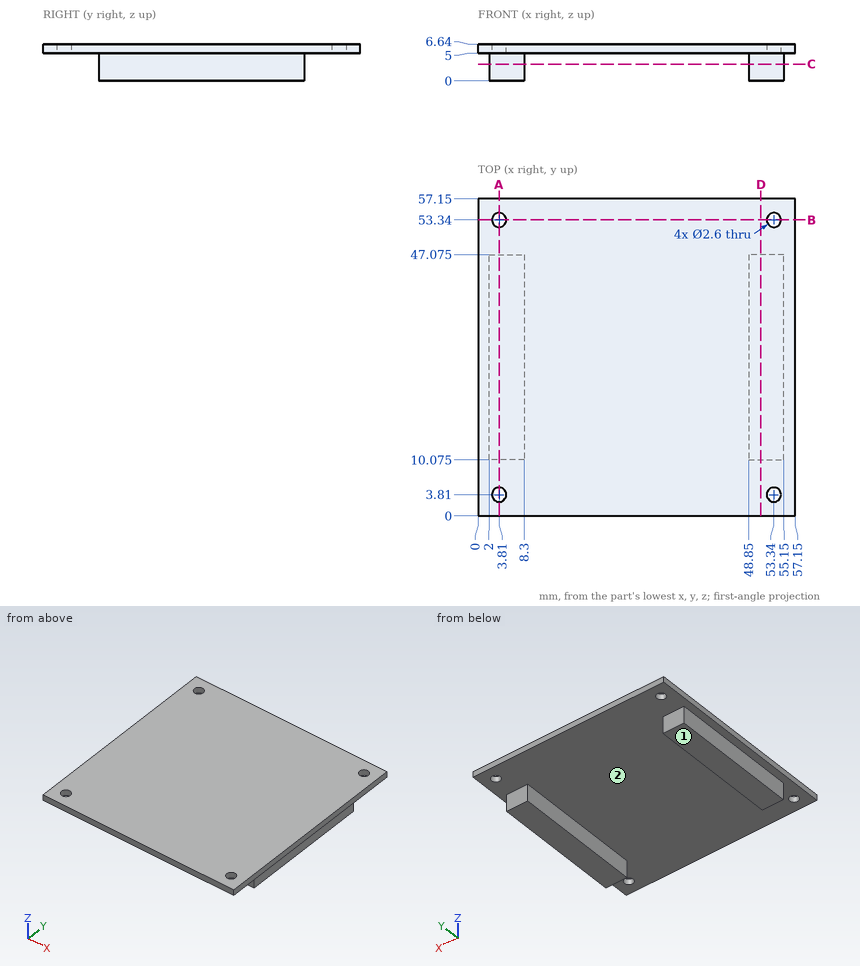
Source: three-view drawing plus pictorial views. Frame: mm from the lowest corner of the part. Round coordinates to 2 decimals unless told otherwise and drop trailing zeros. Loops run counter-clockwise (first coordinate to the right, second up) from the corner with the lowest first, then second, coordinate; pieces in that order, holes last.
1. Ray query, L1, parallel to Y at x = 53.34, z = 6.15; L2, parallel to X at y = 23, z = 3; L3, parallel to Y at x = 54, z = 5.5. Return the intervals inside material, ascending.
2. Section query A-A on x = 3.81. Output: boundary loops of the cut face in (y, z) (3 decimals).
3. Section query B-B on y = 53.34. Output: boundary loops of the cut face in (x, z).
4. Section query C-C on z = 3. Output: boundary loops of the cut face in (x, y) (3 decimals).
5. Contact query for flat-ended pins moving along their axis: pin 1 (2.5 mm diameter, centred on x = 51, z = 3.5, fed in from +Y) (3 decimals); pin 2 (2 mm diameter, centred on y = 40.5, z = 3.5, fed in from +X); pin 3 (2 mm diameter, centred on x = 37, y = 45, fed in from -Z). Output: stop coordinate, or through.
6. Mould query, pull axis X, two halves, no side actions, for the marked faces 1 and 2. Classes: released by +X, released by -X, zero draft, split by the parting line, or undercut.
7. Section query D-D on x = 51. Output: boundary loops of the cut face in (y, z) (3 decimals).
Answers below:
1. L1: y = 0 to 2.51, 5.11 to 52.04, 54.64 to 57.15
1. L2: x = 2 to 8.3, 48.85 to 55.15
1. L3: y = 0 to 2.69, 4.93 to 52.22, 54.46 to 57.15
2. outline: (0, 5) - (2.51, 5) - (2.51, 6.64) - (0, 6.64) - close; (5.11, 5) - (10.075, 5) - (10.075, 0) - (47.075, 0) - (47.075, 5) - (52.04, 5) - (52.04, 6.64) - (5.11, 6.64) - close; (54.64, 5) - (57.15, 5) - (57.15, 6.64) - (54.64, 6.64) - close
3. outline: (0, 5) - (2.51, 5) - (2.51, 6.64) - (0, 6.64) - close; (5.11, 5) - (52.04, 5) - (52.04, 6.64) - (5.11, 6.64) - close; (54.64, 5) - (57.15, 5) - (57.15, 6.64) - (54.64, 6.64) - close
4. outline: (2, 10.075) - (8.3, 10.075) - (8.3, 47.075) - (2, 47.075) - close; (48.85, 10.075) - (55.15, 10.075) - (55.15, 47.075) - (48.85, 47.075) - close
5. pin 1: stops at y = 47.075
5. pin 2: stops at x = 55.15
5. pin 3: stops at z = 5
6. face 1: zero draft
6. face 2: undercut
7. outline: (0, 5) - (10.075, 5) - (10.075, 0) - (47.075, 0) - (47.075, 5) - (57.15, 5) - (57.15, 6.64) - (0, 6.64) - close
